from build123d import *

# Parameters (mm, degrees)
F0_W     = 31.75
F0_H     = 31.75
F1_DEPTH = 31.75
F2_W     = 29.21
F2_H     = 29.21
F3_DEPTH = 31.75
F4_SIZE  = 5.715


with BuildPart() as f1:
    # F0 (on Top) → F1 (new body)
    with BuildSketch(Plane.XY):
        with Locations((15.875, 15.875)):
            Rectangle(F0_W, F0_H)
    extrude(amount=F1_DEPTH)

    # F2 (on face) → F3 (cut, through all)
    with BuildSketch(Plane(origin=(0, 31.75, 0), x_dir=(-1, 0, 0), z_dir=(0, 1, 0))):
        with Locations((-14.605, 17.145)):
            Rectangle(F2_W, F2_H)
    extrude(amount=-F3_DEPTH, mode=Mode.SUBTRACT)

    # F4
    f4_edges = [f1.edges().sort_by_distance(p)[0] for p in [
        (30.48, 31.75, 31.75),
        (30.48, 0, 31.75),
        (0, 0, 1.27),
        (0, 31.75, 1.27),
    ]]
    chamfer(f4_edges, length=F4_SIZE)


solid = f1.part
The model under review builds one solid part; all positions refer to its coordinate system, in mm. A direction names the side the tool comes from. Round coordinates to 2 decimals unless told otherwise and drop trailing zeros. Loops run counter-clockwise (first coordinate to the right, second up) from the corner with the lowest first, then second, coordinate; pieces in that order, holes last. Notation, with made-up numbers: M 16,16.5 L 31,16.5 A15 cw 31,37.5 Z; hole C 12,73.5 d6. An arc over 180 degrees is marked long. Answer as CSV lines item,"result". Start each with the question number.
Item 1: Consider section B-B (y = 16.5). Write out the cut boundary in (x, z).
Item 2: Consider section D-D (z = 21.5). Write out the cut boundary in (x, y), then the cut area to 3 significant figures.
Item 3: Mouldability with a two-part tool opening along Y and no side actions: class faces 3 (the face through (29.21, 16, 17)), 4 (the face through (30.462, 2.898, 28.933)), 5 (the face through (30.462, 28.852, 28.933)) as released by +Y, released by -Y, zero draft, split by the parting line, or undercut.
Item 4: Consider section A-A (z = 2). Write out the cut boundary in (x, y) (3 decimals).
Item 5: Insertion check: P1, Ø14.5, axis at y = 21.5, z = 17, coming from the -X side; P2, Ø9, axis at x = 20.5, y = 14.5, coming from the +Z side; P3, Ø10, axis at x = 11, z = 10.5, coming from the +Y side. Each pin has a flat end and moves straight along its axis. Give the tip position at first contact, or say it passes through.
Item 6: For faces 1 (the face through (15, 16, 2.54)), 2 (the face through (23, 31.75, 2)), list the 3-axis set-ups (+Z, -Z, +X, -X, +Y, -Y) from which the entire face can be reached by the end or side of a thin tool; tool diameter is ignored.
Item 7: Wall thickness on line 1 (X direction, y = 27, z = 17); line 2 (Z direction, x = 29, y = 15); line 3 (Y direction, x = 5, z = 2) (3 decimals): over which ranges is each line inside the solid? List them lowest first. Write a range as [from, to].
Item 8: Consider section C-C (x = 24.5). Write out the cut boundary in (y, z).
Answer:
1,outline,"M 0,0 L 31.75,0 L 31.75,31.75 L 29.21,31.75 L 29.21,2.54 L 0,2.54 Z"
2,outline,"M 29.21,0 L 31.75,0 L 31.75,31.75 L 29.21,31.75 Z"
2,area,"80.6 mm^2"
3,face 3,"zero draft"
3,face 4,"released by -Y"
3,face 5,"released by +Y"
4,outline,"M 0,5.715 L 5.715,0 L 31.75,0 L 31.75,31.75 L 5.715,31.75 L 0,26.035 Z"
5,P1,"stops at x = 29.21"
5,P2,"stops at z = 2.54"
5,P3,"passes through"
6,face 1,"+Z, -X, +Y, -Y"
6,face 2,"+Z, -Z, +X, -X, +Y"
7,line 1,"x = [29.21, 31.75]"
7,line 2,"z = [0, 2.54]"
7,line 3,"y = [0.715, 31.035]"
8,outline,"M 0,0 L 31.75,0 L 31.75,2.54 L 0,2.54 Z"
